from build123d import *

# Parameters (mm, degrees)
PAD001_DEPTH    = 10
PAD002_DEPTH    = 10
SKETCH006_R     = 11
POCKET004_DEPTH = 7
SKETCH007_R     = 4
PAD003_DEPTH    = 7
POCKET005_DEPTH = 24.001
FILLET002_R     = 1
FILLET003_R     = 3
FILLET004_R     = 1


with BuildPart() as part:
    # Sketch004 (on Binder) → Pad001 (new body)
    with BuildSketch(Plane.XY.offset(31)):
        with BuildLine():
            ThreePointArc((11.848552, 14.853007), (-19, 0), (11.848552, -14.853007))
            ThreePointArc((40, -5), (25.087038, -7.534394), (11.848552, -14.853007))
            Line((40, -5), (181, -5))
            Line((181, 5), (181, -5))
            Line((40, 5), (181, 5))
            ThreePointArc((11.848552, 14.853007), (25.087038, 7.534394), (40, 5))
        make_face()
    extrude(amount=PAD001_DEPTH)

    # Sketch005 (on Face7 of Pad001) → Pad002 (join)
    with BuildSketch(Plane(origin=(0, 0, 31), x_dir=(1, 0, 0), z_dir=(0, 0, -1))):
        with BuildLine():
            Line((19, 5), (160, 5))
            ThreePointArc((160, 5), (174.912962, 7.534394), (188.151448, 14.853007))
            ThreePointArc((188.151448, -14.853007), (219, 0), (188.151448, 14.853007))
            ThreePointArc((188.151448, -14.853007), (174.912962, -7.534394), (160, -5))
            Line((160, -5), (19, -5))
            Line((19, -5), (19, 5))
        make_face()
    extrude(amount=PAD002_DEPTH)

    # Sketch006 (on Face7 of Pad002) → Pocket004 (cut)
    with BuildSketch(Plane.XY.offset(31)):
        with Locations((200, 0)):
            Circle(SKETCH006_R)
    extrude(amount=-POCKET004_DEPTH, mode=Mode.SUBTRACT)

    # Sketch007 (on Face4 of Pocket004) → Pad003 (join)
    with BuildSketch(Plane(origin=(0, 0, 31), x_dir=(1, 0, 0), z_dir=(0, 0, -1))):
        Circle(SKETCH007_R)
    extrude(amount=PAD003_DEPTH)

    # Sketch008 (on Face12 of Pad003) → Pocket005 (cut, through all)
    with BuildSketch(Plane.XZ.offset(5)):
        with BuildLine():
            ThreePointArc((89.5, 36.875), (64.835789, 39.966966), (40, 41))
            Line((188.151448, 41), (40, 41))
            Line((188.151448, 31), (188.151448, 41))
            Line((160, 31), (188.151448, 31))
            ThreePointArc((89.5, 36.875), (124.627816, 32.471291), (160, 31))
        make_face()
        with BuildLine():
            ThreePointArc((19, 21), (36.686092, 21.735646), (54.25, 23.9375))
            ThreePointArc((124.75, 23.9375), (89.5, 26.875), (54.25, 23.9375))
            ThreePointArc((124.75, 23.9375), (142.313908, 21.735646), (160, 21))
            Line((19, 21), (160, 21))
        make_face()
    extrude(amount=-POCKET005_DEPTH, mode=Mode.SUBTRACT)

    # Fillet002
    fillet002_edges = [part.edges().sort_by_distance(p)[0] for p in [
        (-4, 0, 24),
    ]]
    fillet(fillet002_edges, radius=FILLET002_R)

    # Fillet003
    fillet003_edges = [part.edges().sort_by_distance(p)[0] for p in [
        (19, 5, 26),
        (19, -5, 26),
    ]]
    fillet(fillet003_edges, radius=FILLET003_R)

    # Fillet004
    fillet004_edges = [part.edges().sort_by_distance(p)[0] for p in [
        (219, 0, 21),
        (-19, 0, 41),
    ]]
    fillet(fillet004_edges, radius=FILLET004_R)


solid = part.part
Geometry check sheet. Reference: the model listing, model coordinates, mm. A direction names the side the tool comes from. Give positions to 0.01 mm unless a question says otherwise; leave off trailing zeros. Answer as a JSON object with one key per item and string values.
(1) Draft check along Y on faces 1 (the flat face through (200, 0, 24)), 2 (the cylindrical face through (65.18, -0.06, 39.94)), 3 (the cylindrical face through (189, 0, 28)), 4 (the cylindrical face through (174.712, -7.465, 26.056)). Enter one of: released by +Y, released by -Y, zero draft, split by the parting line, or undercut.
Report:
{"face 1": "undercut", "face 2": "zero draft", "face 3": "undercut", "face 4": "released by -Y"}
(2) Depth check by flat-ended pin: pin 1 Ø4 at (x, y) = (103.5, 0) entering from -Z; pin 2 Ø6 at (x, z) = (12, 25.5) entering from +Y; pin 3 Ø17.5 at (x, y) = (195.5, 4.5) entering from +Z; pin 4 Ø9 at (x, z) = (86, 35) entering from -Y. Enter the tip coordinate at first touch or a pass-through.
Report:
{"pin 1": "z = 26.27", "pin 2": "through", "pin 3": "z = 31", "pin 4": "y = -5"}
(3) Tool access check on faces 5 (the flat face through (0, 0, 24)), 6 (the cylindrical face through (36.947, -0.056, 21.758)), 7 (the flat face through (188.6, -0.3, 31)). Record the directions out of +Z, -Z, +X, -X, +Y, -Y that give a thin tool (end or side, any length) a straight path to the whole face; none if there is none.
Report:
{"face 5": "-Z, -X, +Y, -Y", "face 6": "-Z, +Y, -Y", "face 7": "+Z, +X, +Y, -Y"}
(4) Material ranges on line 1 (Y direction, x = 200, z = 28.5); line 2 (X direction, y = 3, z = 30); line 3 (Z direction, x = 206, y = 15), recorded low to high.
Report:
{"line 1": "-19 to -11, 11 to 19", "line 2": "-2.65 to 2.65, 19.17 to 189.42, 210.58 to 218.76", "line 3": "21 to 31"}
